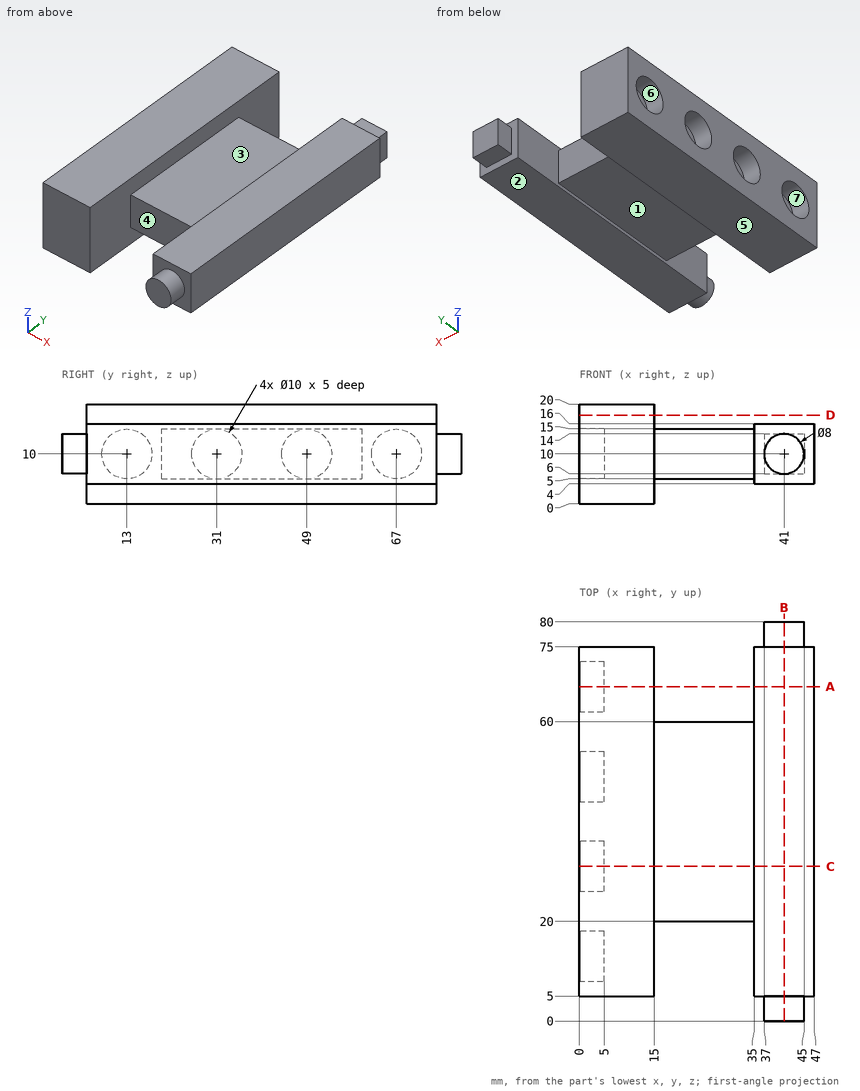
For this review, use the dimensioned drawing (mm, ordinates from the lowest corner) and the shaded views. A direction names the side the tool comes from. Give positions to 0.01 mm unless a question says otherwise; leave off trailing zeros. Order: outer loops, then holes, each group sorted by start corner. A loop starts at its lowest first (then second) coordinate and runs counter-clockwise, first axis right, second up. Notation, with made-up numbers: (-34, 34.5) - (-30, 34.5) arc R18 cw to (-30, 50.5) - close; hole circle Ø6 at (28, 69). An arc over 180 degrees is marked (long way). Use a Markdown table: item, result. Add a question column.
(1) Add section C-C on y = 31. Give the boundary of the cut face in (x, z).
(2) Wall thickness on probe 1 along Z at (x, y) = (1.1, 13); probe 2 along X at (y, z) = (17, 8); probe 3 along X at (y, z) = (64, 5.5): over which ranges is each line inside the solid? List them lowest first. Write a range as [from, to].
(3) Add section D-D on z = 17.75. Give the boundary of the cut face in (x, y).
(4) Machinability: for the marked faces 1, 2 and 3, which of the approach directions +Z, -Z, +X, -X, +Y, -Y give a long, thin tool a straight path to every point of the face, cutting with its end or side? Answer none if there is none.
(5) Add section A-A on y = 67. Give the boundary of the cut face in (x, z), then the cut area to 3 significant figures.
(6) Add section B-B on x = 41. Give the boundary of the cut face in (y, z), then the cut area to 3 significant figures.
(7) Clearance check with flat-ended pins moving along their axes: P1, Ø5.5, axis at x = 41.5, y = 76.5, coming from the +Z side; P2, Ø4, axis at y = 78, z = 10, coming from the +X side; P3, Ø6, axis at x = 40.5, z = 10.5, coming from the -Y side; P4, Ø8, axis at y = 31, z = 10.5, coming from the -X side. State where each tip first meets the part, or that it passes through.
(8) Mouldability with a two-part tool opening along Y and no side actions: class the marked faces 4, 5, 6 and 7 as +Y half, -Y half, draft (parallel to the pull), parting line (faces both ways), or undercut.
Report:
| question | item | result |
|---|---|---|
| 1 | outline | (0, 0) - (15, 0) - (15, 5) - (35, 5) - (35, 4) - (47, 4) - (47, 16) - (35, 16) - (35, 15) - (15, 15) - (15, 20) - (0, 20) - (0, 15) - (5, 15) - (5, 5) - (0, 5) - close |
| 2 | probe 1 | z = [0, 5], [15, 20] |
| 2 | probe 2 | x = [5, 15], [35, 47] |
| 2 | probe 3 | x = [0, 15], [35, 47] |
| 3 | outline | (0, 5) - (15, 5) - (15, 75) - (0, 75) - close |
| 4 | face 1 | -Z, +Y, -Y |
| 4 | face 2 | -Z, +X, +Y, -Y |
| 4 | face 3 | +Z, +Y, -Y |
| 5 | outline | (0, 0) - (15, 0) - (15, 20) - (0, 20) - (0, 15) - (5, 15) - (5, 5) - (0, 5) - close; (35, 4) - (47, 4) - (47, 16) - (35, 16) - close |
| 5 | area | 394 mm² |
| 6 | outline | (0, 6) - (5, 6) - (5, 4) - (75, 4) - (75, 6) - (80, 6) - (80, 14) - (75, 14) - (75, 16) - (5, 16) - (5, 14) - (0, 14) - close |
| 6 | area | 920 mm² |
| 7 | P1 | stops at z = 16 |
| 7 | P2 | stops at x = 45 |
| 7 | P3 | stops at y = 0 |
| 7 | P4 | stops at x = 5 |
| 8 | face 4 | -Y half |
| 8 | face 5 | draft |
| 8 | face 6 | undercut |
| 8 | face 7 | undercut |
